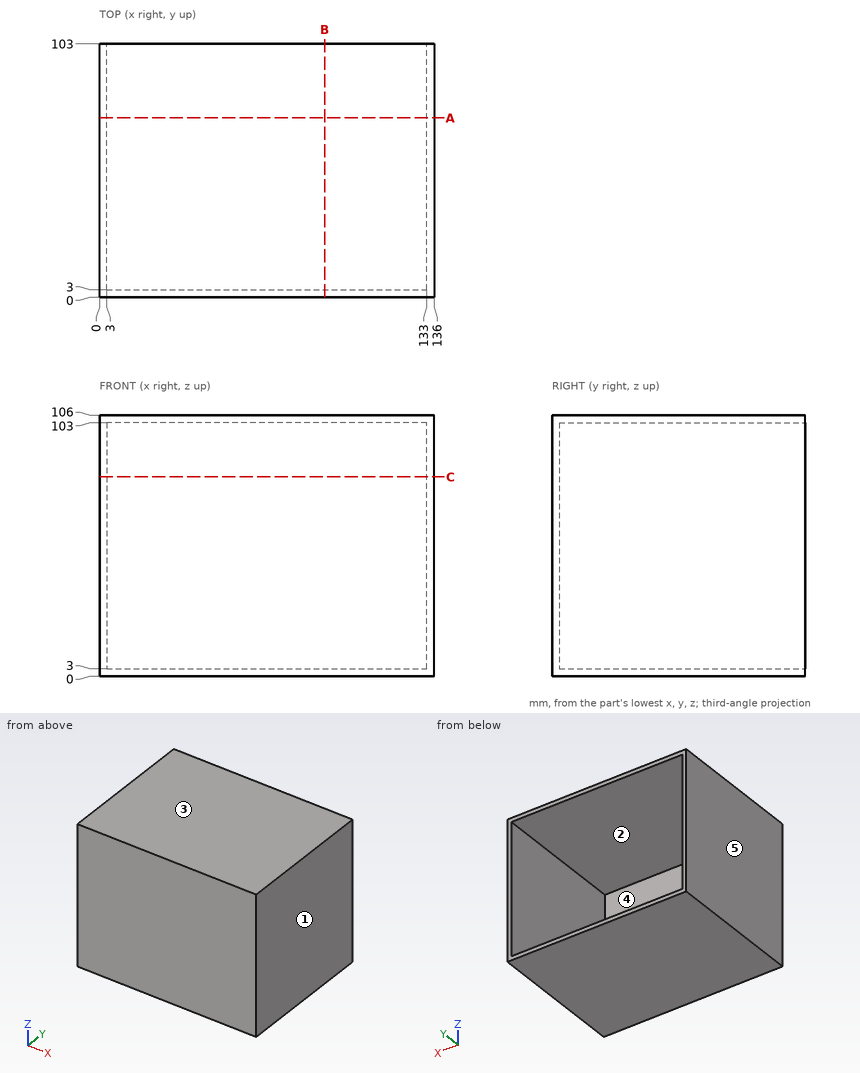
Geometry check sheet. Reference: drawing and pictorial views, mm from the part's lowest x, y, z. A direction names the side the tool comes from. Coordinates: 2 decimals unless noted, no trailing zeros. Write each loop counter-clockwise with the first axis right and the second up, starting at its lowest first coordinate (ties: lowest second). Pieces come first, ordered by that corner, then holes. Notation, with made-up numbers: M -21,18.5 L 7,18.5 A25 ccw 7,51.5 Z; hole C 54.25,-19.5 d6. An arc over 180 degrees is marked long. One line per question, with ' | ' between items.
1) Sectioned sample at B-B on x = 91.5. Record the cut outline in (y, z), then the cut area to 3 significant figures.
Solutions:
outline: M 0,0 L 103,0 L 103,3 L 3,3 L 3,103 L 103,103 L 103,106 L 0,106 Z | area: 918 mm^2
2) Release check for a two-part mould opening along Z. For the marked faces 3, 4 and 5 record: +Z half, -Z half, draft (parallel to the pull), parting line (faces both ways), or undercut.
Solutions:
face 3: +Z half | face 4: undercut | face 5: draft
3) Depth check by flat-ended pin: pin 1 Ø1 at (y, z) = (18.5, 14.5) entering from -X; pin 2 Ø2 at (x, z) = (22, 52.5) entering from +Y. Enter the tip coordinate at first touch or a pass-through.
Solutions:
pin 1: x = 0 | pin 2: y = 3
4) Material ranges on L1, parallel to Z at x = 59.5, y = 49.5; L2, parallel to X at y = 68.5, z = 56.5; L3, parallel to Y at x = 65, z = 49, recorded low to high.
Solutions:
L1: 0 to 3, 103 to 106 | L2: 0 to 3, 133 to 136 | L3: 0 to 3
5) Sectioned sample at A-A on y = 73. Record the cut outline in (x, z), then the cut area to 3 significant figures.
Solutions:
outline: M 0,0 L 136,0 L 136,106 L 0,106 Z; hole M 3,3 L 133,3 L 133,103 L 3,103 Z | area: 1,420 mm^2
6) Sectioned sample at C-C on z = 81. Record the cut outline in (x, y).
Solutions:
outline: M 0,0 L 136,0 L 136,103 L 133,103 L 133,3 L 3,3 L 3,103 L 0,103 Z
7) Access from +Z, -Z, +X, -X, +Y, -Y to the whole of each face (thin tool, end or side, straight path). Record for the marked faces 1 and 2.
Solutions:
face 1: +Z, -Z, +X, +Y, -Y | face 2: +Y
